```python
from build123d import *

# Parameters (mm, degrees)
BOSS_EXTRUDE1_DEPTH       = 50.8
SHELL1_T                  = -2.54
SKETCH2_W                 = 45.72
SKETCH2_H                 = 45.72
CUT_EXTRUDE2_DEPTH        = 50.8
F_97_0_5_DIAMETER_HOLE1_D = 12.7
F_97_0_5_DIAMETER_HOLE2_D = 12.7
F_97_0_5_DIAMETER_HOLE3_D = 12.7


with BuildPart() as part:
    # Sketch1 → Boss-Extrude1 (new body)
    with BuildSketch(Plane.XY):
        with BuildLine():
            Line((0, 1057.275), (0, 50.8))
            ThreePointArc((0, 50.8), (14.878975516, 14.878975516), (50.8, 0))
            Line((50.8, 0), (384.175, 0))
            Line((384.175, 0), (384.175, 50.8))
            Line((384.175, 50.8), (101.6, 50.8))
            ThreePointArc((101.6, 50.8), (65.678975516, 65.678975516), (50.8, 101.6))
            Line((50.8, 101.6), (50.8, 1057.275))
            Line((50.8, 1057.275), (0, 1057.275))
        make_face()
    extrude(amount=BOSS_EXTRUDE1_DEPTH)

    # Shell1
    shell1_openings = [part.faces().sort_by_distance(p)[0] for p in [
        (25.4, 1057.275, 25.4),
    ]]
    offset(amount=SHELL1_T, openings=shell1_openings, kind=Kind.INTERSECTION)

    # Sketch2 → Cut-Extrude2 (cut)
    with BuildSketch(Plane(origin=(384.175, 0, 0), x_dir=(0, 0, -1), z_dir=(1, 0, 0))):
        with Locations((-25.4, 25.4)):
            Rectangle(SKETCH2_W, SKETCH2_H)
    extrude(amount=-CUT_EXTRUDE2_DEPTH, mode=Mode.SUBTRACT)

    # #97 (0.5) Diameter Hole1 (through all)
    with Locations(Plane(origin=(365.125, 25.4, 50.8), x_dir=(1, 0, 0), z_dir=(0, 0, 1))):
        with Locations((0, 0), (-146.05, 0)):
            Hole(F_97_0_5_DIAMETER_HOLE1_D / 2)

    # #97 (0.5) Diameter Hole2 (through all)
    with Locations(Plane(origin=(0, 1031.875, 25.4), x_dir=(0, 0, -1), z_dir=(-1, 0, 0))):
        with Locations((0, 0)):
            Hole(F_97_0_5_DIAMETER_HOLE2_D / 2)

    # #97 (0.5) Diameter Hole3 (through all)
    with Locations(Plane(origin=(25.4, 968.375, 50.8), x_dir=(1, 0, 0), z_dir=(0, 0, 1))):
        with Locations((0, 0)):
            Hole(F_97_0_5_DIAMETER_HOLE3_D / 2)


solid = part.part
```
Design review of the part built by this model. Coordinates are the model's own, in mm. A direction names the side the tool comes from. Give positions to 0.01 mm unless a question says otherwise; leave off trailing zeros. Order: outer loops, then holes, each group sorted by start corner. A loop starts at its lowest first (then second) coordinate and runs counter-clockwise, first axis right, second up. Notation, with made-up numbers: (14.25, 66.25) -> (38.25, 66.25) arc R8 ccw to (38.25, 77.25) -> close; hole circle Ø8 at (27.25, -30). An arc over 180 degrees is marked (long way). Write each question's results on one line, items separated by ' | '. Start each with the question number.
Q1. Wall thickness on L1, parallel to Z at x = 31, y = 141.5: over which ranges is the line inside the solid? List them lowest first. Write a range as from..to.
Q2. For pin 1 (20.5 mm diameter, centred on y = 1031.875, z = 25.4, fed in from -X); pin 2 (15 mm diameter, centred on x = 262.5, z = 17, fed in from +Y); pin 3 (13.5 mm diameter, centred on y = 776, z = 21, fed in from +X); pin 4 (2 mm diameter, centred on x = 91.5, z = 6, fed in from +Y), all flat-tipped, find the tip position at first contact; note any pin that passes through.
Q3. Machinability: for faces 4 (the flat face through (245, 50.8, 25)), 5 (the flat face through (48.26, 573, 25)), 6 (the flat face through (215, 2.54, 25)), 7 (the flat face through (37, 415, 48.26)), 8 (the flat face through (215, 0, 25)), which of the approach directions +Z, -Z, +X, -X, +Y, -Y give a long, thin tool a straight path to every point of the face, cutting with its end or side? Answer none if there is none.
Q4. Add section B-B on z = 40. Give the boundary of the cut face in (x, y) (3 decimals).
Q5. Mouldability with a two-part tool opening along Y and no side actions: class faces 1 (the flat face through (50.8, 573, 25)), 2 (the flat face through (27, 1057.275, 50)), 3 (the flat face through (245, 48.26, 25)) as +Y half, -Y half, draft (parallel to the pull), parting line (faces both ways), or undercut.
Q6. Add section A-A on x = 171.5. Give the boundary of the cut face in (y, z).
Found:
1) L1: z = 0..2.54, 48.26..50.8
2) pin 1: stops at x = 0 | pin 2: stops at y = 50.8 | pin 3: stops at x = 50.8 | pin 4: stops at y = 52.03
3) face 4: +Z, -Z, +X, +Y | face 5: +Y | face 6: +X | face 7: none | face 8: +Z, -Z, +X, -X, -Y
4) outline: (0, 50.8) arc R50.8 ccw to (50.8, 0) -> (384.175, 0) -> (384.175, 2.54) -> (50.8, 2.54) arc R48.26 cw to (2.54, 50.8) -> (2.54, 1057.275) -> (0, 1057.275) -> close; (48.26, 101.6) arc R53.34 ccw to (101.6, 48.26) -> (384.175, 48.26) -> (384.175, 50.8) -> (101.6, 50.8) arc R50.8 cw to (50.8, 101.6) -> (50.8, 1057.275) -> (48.26, 1057.275) -> close
5) face 1: draft | face 2: +Y half | face 3: undercut
6) outline: (0, 0) -> (50.8, 0) -> (50.8, 50.8) -> (0, 50.8) -> close; hole (2.54, 2.54) -> (48.26, 2.54) -> (48.26, 48.26) -> (2.54, 48.26) -> close
